Study the drawing (mm; zero at the part's minimum x, y, z) and answer. A direction names the side the tool comes from. Give positions to 0.01 mm unless a question says otherwise; leave off trailing zeros. Loops run counter-clockwise (first coordinate to the right, second up) from the corner with the lowest first, then second, coordinate; pieces in that order, holes last. Notation, with made-up numbers: (83.5, -17) - (97.5, -17) arc R29 ccw to (97.5, 14) - close; hole circle Ø3 at (85.5, 69.5). An arc over 180 degrees is marked (long way). One line per item, written item: value. Start each with the question number.
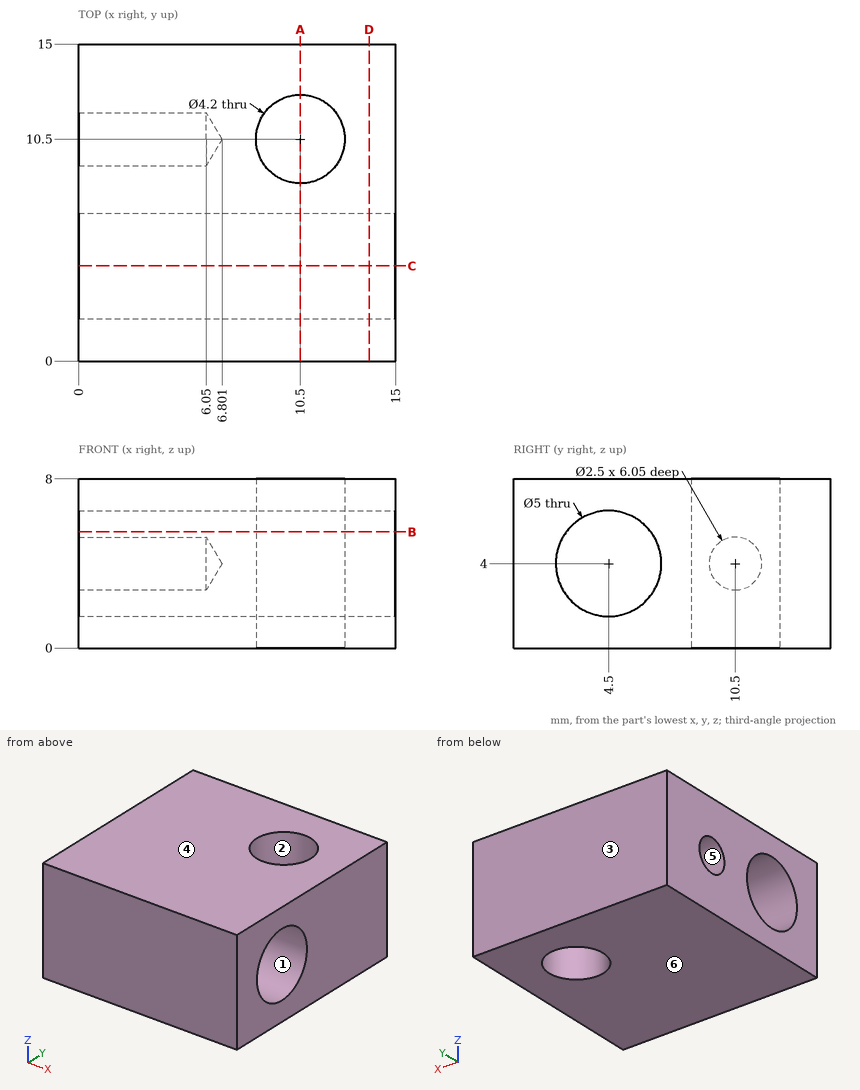
1. A cutting plane is placed at B-B (z = 5.5). Determine the outline of the cut face in (x, y).
2. A flat-ended cylindrical pin translates along its axis: pin 1 (4 mm diameter, centred on y = 4.5, z = 4, fed in from +X). Find the tip coordinate at first contact, or state that the pin passes through.
3. A cutting plane is placed at D-D (x = 13.75). Determine the outline of the cut face in (y, z), plus the area to 3 significant figures.
4. Find the intervals of material crossed by L1, parallel to Y at x = 2, z = 4; L2, parallel to Z at x = 2.5, y = 10.5; L3, parallel to Y at x = 7.5, z = 4, in increasing order. Write a range as [from, to].
5. A cutting plane is placed at C-C (y = 4.5). Determine the outline of the cut face in (x, z), plus the area to 3 significant figures.
6. For the marked faces 5 and 6, determine the directions among +Z, -Z, +X, -X, +Y, -Y from which every point of the face is accessible in a straight line to the end or side of a thin tool.
7. A cutting plane is placed at A-A (x = 10.5). Determine the outline of the cut face in (y, z).
8. Determine the mould class of the marked faces 1, 2, 3 and 4 for opening direction Y: released by +Y, released by -Y, zero draft, split by the parting line, or undercut.
Results below:
1. outline: (0, 0) - (15, 0) - (15, 2.5) - (0, 2.5) - close; (0, 6.5) - (15, 6.5) - (15, 15) - (0, 15) - close; hole circle Ø4.2 at (10.5, 10.5)
2. pin 1: passes through
3. outline: (0, 0) - (15, 0) - (15, 8) - (0, 8) - close; hole circle Ø5 at (4.5, 4)
3. area: 100 mm^2
4. L1: y = [0, 2], [7, 9.25], [11.75, 15]
4. L2: z = [0, 2.75], [5.25, 8]
4. L3: y = [0, 2], [7, 15]
5. outline: (0, 0) - (15, 0) - (15, 1.5) - (0, 1.5) - close; (0, 6.5) - (15, 6.5) - (15, 8) - (0, 8) - close
5. area: 45.0 mm^2
6. face 5: -X
6. face 6: -Z, +X, -X, +Y, -Y
7. outline: (0, 0) - (8.4, 0) - (8.4, 8) - (0, 8) - close; (12.6, 0) - (15, 0) - (15, 8) - (12.6, 8) - close; hole circle Ø5 at (4.5, 4)
8. face 1: undercut
8. face 2: undercut
8. face 3: released by +Y
8. face 4: zero draft
